```python
from build123d import *

# Parameters (mm, degrees)
SKETCH1_W           = 70
SKETCH1_H           = 65
SKETCH1_R           = 2.5
BOSS_EXTRUDE1_DEPTH = 5
FILLET1_R           = 10
SKETCH2_W           = 70
SKETCH2_H           = 24
BOSS_EXTRUDE2_DEPTH = 25
FILLET2_R           = 2.5
SKETCH3_R           = 5
SKETCH3_R_2         = 7.5
CUT_EXTRUDE1_DEPTH  = 30
SKETCH4_R           = 1.75
CUT_EXTRUDE2_DEPTH  = 30
FILLET3_R           = 2.5
SKETCH6_W           = 8.533797122
SKETCH6_H           = 2.5
SKETCH6_W_2         = 12.888873946
CUT_EXTRUDE3_DEPTH  = 30


with BuildPart() as part:
    # Sketch1 → Boss-Extrude1 (new body)
    with BuildSketch(Plane.XY):
        with Locations((-15.487804878, -14.329268293)):
            Rectangle(SKETCH1_W, SKETCH1_H)
        with Locations((-42.987804878, 10.670731707)):
            Circle(SKETCH1_R, mode=Mode.SUBTRACT)
        with Locations((12.012195122, 10.670731707)):
            Circle(SKETCH1_R, mode=Mode.SUBTRACT)
        with Locations((-42.987804878, -39.329268293)):
            Circle(SKETCH1_R, mode=Mode.SUBTRACT)
        with Locations((12.012195122, -39.329268293)):
            Circle(SKETCH1_R, mode=Mode.SUBTRACT)
    extrude(amount=BOSS_EXTRUDE1_DEPTH)

    # Fillet1
    fillet1_edges = [part.edges().sort_by_distance(p)[0] for p in [
        (-50.487804878, 18.170731707, 2.5),
        (19.512195122, 18.170731707, 2.5),
        (19.512195122, -46.829268293, 2.5),
        (-50.487804878, -46.829268293, 2.5),
    ]]
    fillet(fillet1_edges, radius=FILLET1_R)

    # Sketch2 → Boss-Extrude2 (add)
    with BuildSketch(Plane.XY.offset(5)):
        with Locations((-15.487804878, -14.329268293)):
            Rectangle(SKETCH2_W, SKETCH2_H)
    extrude(amount=BOSS_EXTRUDE2_DEPTH)

    # Fillet2
    fillet2_edges = [part.edges().sort_by_distance(p)[0] for p in [
        (-15.487804878, -26.329268293, 5),
        (-15.487804878, -2.329268293, 5),
    ]]
    fillet(fillet2_edges, radius=FILLET2_R)

    # Sketch3 → Cut-Extrude1 (cut)
    with BuildSketch(Plane(origin=(0, -2.329268293, 0), x_dir=(1, 0, 0), z_dir=(0, 1, 0))):
        with Locations(Location((-15.487804878, -18.75, 0), (0, 0, 180))):
            Circle(SKETCH3_R)
        with Locations(Location((-40.487804878, -18.75, 0), (0, 0, 180))):
            Circle(SKETCH3_R_2)
        with Locations(Location((9.512195122, -18.75, 0), (0, 0, 180))):
            Circle(SKETCH3_R_2)
    extrude(amount=-CUT_EXTRUDE1_DEPTH, mode=Mode.SUBTRACT)

    # Sketch4 → Cut-Extrude2 (cut)
    with BuildSketch(Plane(origin=(0, -2.329268293, 0), x_dir=(1, 0, 0), z_dir=(0, 1, 0))):
        with Locations(Location((-21.144659128, -13.093145751, 0), (0, 0, 180))):
            Circle(SKETCH4_R)
        with Locations(Location((-9.830950629, -13.093145751, 0), (0, 0, 180))):
            Circle(SKETCH4_R)
        with Locations(Location((-9.830950629, -24.406854249, 0), (0, 0, 180))):
            Circle(SKETCH4_R)
        with Locations(Location((-21.144659128, -24.406854249, 0), (0, 0, 180))):
            Circle(SKETCH4_R)
    extrude(amount=-CUT_EXTRUDE2_DEPTH, mode=Mode.SUBTRACT)

    # Fillet3
    fillet3_edges = [part.edges().sort_by_distance(p)[0] for p in [
        (-50.487804878, -14.329268293, 30),
        (19.512195122, -14.329268293, 30),
    ]]
    fillet(fillet3_edges, radius=FILLET3_R)

    # Sketch6 → Cut-Extrude3 (cut)
    with BuildSketch(Plane(origin=(0, -2.329268293, 0), x_dir=(1, 0, 0), z_dir=(0, 1, 0))):
        with Locations((-47.987804878, -18.75)):
            Rectangle(SKETCH6_W, SKETCH6_H)
        with Locations((17.012195122, -18.75)):
            Rectangle(SKETCH6_W_2, SKETCH6_H)
    extrude(amount=-CUT_EXTRUDE3_DEPTH, mode=Mode.SUBTRACT)


solid = part.part
```
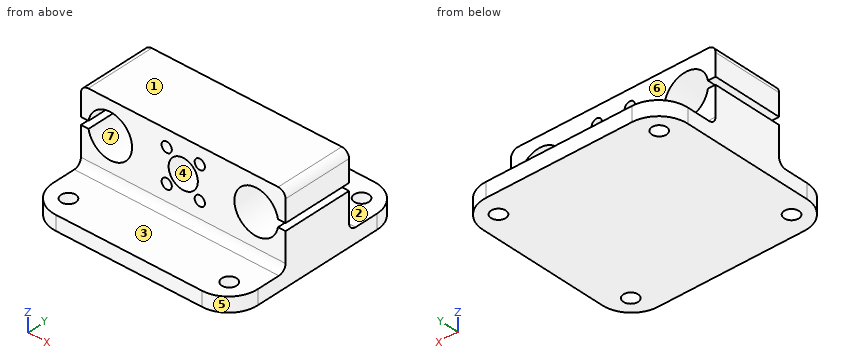
Work out the finished part from the listing and answer in its coordinate system (mm). Face numbers are marked on the shaded views. A direction names the side the tool comes from. Give positions to 0.01 mm unless a question says otherwise; leave off trailing zeros. Loops run counter-clockwise (first coordinate to the right, second up) from the corner with the lowest first, then second, coordinate; pieces in that order, holes last. Notation, with made-up numbers: (27.25, 83) -> (33.25, 83) arc R19 ccw to (33.25, 101) -> close; hole circle Ø5 at (-2.75, -26). An arc over 180 degrees is marked (long way). Write item = value, one per line. Start each with the question number.
(1) The mould has two halves that part along X. Classify the marked faces 4, 5, 6 and 7: +X half, -X half, draft (parallel to the pull), parting line (faces both ways), or undercut.
(2) Find section C-C on y = -11.5. Give the vertices of the cut face in (x, z).
(3) Given pin 1 Ø4 at (x, y) = (-12, -35) entering from +Z; pin 2 Ø10 at (x, z) = (-1, 23) entering from +Y; pin 3 Ø13.5 at (x, z) = (9.51, 18.75) entering from -Y; pin 4 Ø4.5 at (x, z) = (-9.83, 24.41) entering from -Y, each flat-ended and moving along its own axis, determine where each tip first touches the part or whether it passes through.
(4) Which of the six approach directions +Z, -Z, +X, -X, +Y, -Y give full straight-line access (tool end or side, diameter ignored) to the marked faces 1, 2 and 3?
(5) Find section D-D on x = -38.5. Give the vertices of the cut face in (y, z).
(6) Find section B-B on x = -1. Give the vertices of the cut face in (y, z), and give its area (3 significant figures).
(7) Find the intervals of material crossed by probe 1 along Z at (x, y) = (-5.5, 9.5); probe 2 along Y at (x, z) = (-30, 16.25); probe 3 along Z at (x, y) = (-17, -9.5), in increasing order. Write a range as from..to.
(8) Find section A-A on z = 18.75. Give the vertices of the cut face in (x, y).
From the geometry:
q1.face_4 = undercut
q1.face_5 = +X half
q1.face_6 = draft
q1.face_7 = undercut
q2.outline = (-50.49, 0) -> (19.51, 0) -> (19.51, 17.5) -> (16.91, 17.5) arc R7.5 cw (long way) to (16.91, 20) -> (19.51, 20) -> (19.51, 27.5) arc R2.5 ccw to (17.01, 30) -> (-47.99, 30) arc R2.5 ccw to (-50.49, 27.5) -> (-50.49, 20) -> (-47.88, 20) arc R7.5 cw (long way) to (-47.88, 17.5) -> (-50.49, 17.5) -> close; hole circle Ø3.5 at (-21.14, 13.09); hole circle Ø3.5 at (-21.14, 24.41); hole circle Ø10 at (-15.49, 18.75); hole circle Ø3.5 at (-9.83, 13.09); hole circle Ø3.5 at (-9.83, 24.41)
q3.pin_1 = 5
q3.pin_2 = -2.33
q3.pin_3 = through
q3.pin_4 = -26.33
q4.face_1 = +Z, +X, -X, +Y, -Y
q4.face_2 = +Z, +X, -X, +Y
q4.face_3 = +Z, +X, -X, -Y
q5.outline = (-46.83, 0) -> (18.17, 0) -> (18.17, 5) -> (0.17, 5) arc R2.5 cw to (-2.33, 7.5) -> (-2.33, 11.52) -> (-26.33, 11.52) -> (-26.33, 7.5) arc R2.5 cw to (-28.83, 5) -> (-46.83, 5) -> close; (-26.33, 25.98) -> (-2.33, 25.98) -> (-2.33, 30) -> (-26.33, 30) -> close
q6.outline = (-46.83, 0) -> (18.17, 0) -> (18.17, 5) -> (0.17, 5) arc R2.5 cw to (-2.33, 7.5) -> (-2.33, 30) -> (-26.33, 30) -> (-26.33, 7.5) arc R2.5 cw to (-28.83, 5) -> (-46.83, 5) -> close
q6.area = 928 mm^2
q7.probe_1 = 0..5
q7.probe_2 = -26.33..-2.33
q7.probe_3 = 0..13.98, 23.52..30
q8.outline = (-32.99, -26.33) -> (-20.49, -26.33) -> (-20.49, -2.33) -> (-32.99, -2.33) -> close; (-10.49, -26.33) -> (2.01, -26.33) -> (2.01, -2.33) -> (-10.49, -2.33) -> close
